from build123d import *

# Parameters (mm, degrees)
BOSS_EXTRUDE1_DEPTH            = 100
CUT_EXTRUDE3_DEPTH             = 202.556443707
CUT_EXTRUDE3_DEPTH_BACK        = 202.556443707
SKETCH4_4_R                    = 9.85
CUT_EXTRUDE4_DEPTH             = 3
CUT_EXTRUDE5_START             = 103
SKETCH4_6_R                    = 9.85
CUT_EXTRUDE5_DEPTH             = 103
CUT_EXTRUDE6_REACH             = 206.206
SKETCH5_R                      = 2.25
CUT_EXTRUDE6_DIRECTION_2_DEPTH = 205.205778567
CUT_EXTRUDE7_REACH             = 201.841
SKETCH6_R                      = 2.25
SKETCH7_W                      = 12
SKETCH7_H                      = 15
CUT_EXTRUDE8_DEPTH             = 197.242821038
FILLET3_R                      = 2.5
FILLET4_R                      = 2.5
FILLET6_R                      = 5
CUT_EXTRUDE11_REACH            = 198.243
SKETCH8_W                      = 41.5
SKETCH8_H                      = 5
CUT_EXTRUDE12_REACH            = 174.119
SKETCH9_R                      = 1.75


with BuildPart() as part:
    # Sketch1 → Boss-Extrude1 (new body)
    with BuildSketch(Plane.XY):
        Polygon((-10.600610125, 140), (-15.600610125, 140), (-15.600610125, -5), (94.399389875, -5), (94.399389875, 140), (89.399389875, 140), (89.399389875, 0), (-10.600610125, 0), align=None)
    extrude(amount=-BOSS_EXTRUDE1_DEPTH)

    # Sketch4 → Cut-Extrude3 (cut, two sides: drawn at the far end of the back side and taken through both)
    with BuildSketch(Plane.ZY.offset(-89.399389875).offset(-CUT_EXTRUDE3_DEPTH_BACK)):
        with BuildLine():
            ThreePointArc((-89.05, 45), (-82.05, 38), (-75.05, 45))
            Line((-75.05, 45), (-82.05, 45))
            Line((-82.05, 45), (-89.05, 45))
        make_face()
        with BuildLine():
            Line((-82.05, 45), (-75.05, 45))
            ThreePointArc((-75.05, 45), (-82.05, 52), (-89.05, 45))
            Line((-89.05, 45), (-82.05, 45))
        make_face()
        with BuildLine():
            ThreePointArc((-57, 45), (-50, 38), (-43, 45))
            Line((-43, 45), (-50, 45))
            Line((-50, 45), (-57, 45))
        make_face()
        with BuildLine():
            Line((-50, 45), (-43, 45))
            ThreePointArc((-43, 45), (-50, 52), (-57, 45))
            Line((-57, 45), (-50, 45))
        make_face()
        with BuildLine():
            ThreePointArc((-24.95, 45), (-17.95, 38), (-10.95, 45))
            Line((-10.95, 45), (-17.95, 45))
            Line((-17.95, 45), (-24.95, 45))
        make_face()
        with BuildLine():
            Line((-17.95, 45), (-10.95, 45))
            ThreePointArc((-10.95, 45), (-17.95, 52), (-24.95, 45))
            Line((-24.95, 45), (-17.95, 45))
        make_face()
    extrude(amount=CUT_EXTRUDE3_DEPTH + CUT_EXTRUDE3_DEPTH_BACK, mode=Mode.SUBTRACT)

    # Sketch4<4> → Cut-Extrude4 (cut)
    with BuildSketch(Plane.ZY.offset(-89.399389875)):
        with Locations((-50, 45)):
            Circle(SKETCH4_4_R)
        with Locations((-82.05, 45)):
            Circle(SKETCH4_4_R)
        with Locations((-17.95, 45)):
            Circle(SKETCH4_4_R)
    extrude(amount=-CUT_EXTRUDE4_DEPTH, mode=Mode.SUBTRACT)

    # Sketch4<6> → Cut-Extrude5 (cut)
    with BuildSketch(Plane.ZY.offset(-89.399389875).offset(CUT_EXTRUDE5_START)):
        with Locations((-50, 45)):
            Circle(SKETCH4_6_R)
        with Locations((-82.05, 45)):
            Circle(SKETCH4_6_R)
        with Locations((-17.95, 45)):
            Circle(SKETCH4_6_R)
    extrude(amount=-CUT_EXTRUDE5_DEPTH, mode=Mode.SUBTRACT)

    # Sketch5 → Cut-Extrude6 (cut, up to next)
    with BuildSketch(Plane.ZY.offset(15.600610125), mode=Mode.PRIVATE) as cut_extrude6_sk1:
        with Locations(Location((-78.75, 119.5, 0), (0, 0, 90))):
            Circle(SKETCH5_R)
    cut_extrude6_tool1 = extrude(cut_extrude6_sk1.sketch, amount=-CUT_EXTRUDE6_REACH, mode=Mode.PRIVATE) & part.part
    # Sketch5 → Cut-Extrude6 (cut, up to next)
    with BuildSketch(Plane.ZY.offset(15.600610125), mode=Mode.PRIVATE) as cut_extrude6_sk2:
        with Locations(Location((-21.25, 119.5, 0), (0, 0, 90))):
            Circle(SKETCH5_R)
    cut_extrude6_tool2 = extrude(cut_extrude6_sk2.sketch, amount=-CUT_EXTRUDE6_REACH, mode=Mode.PRIVATE) & part.part
    add(cut_extrude6_tool1.solids().sort_by_distance((-15.60061, 119.5, -78.75))[0], mode=Mode.SUBTRACT)
    add(cut_extrude6_tool2.solids().sort_by_distance((-15.60061, 119.5, -21.25))[0], mode=Mode.SUBTRACT)

    # Sketch5 → Cut-Extrude6 direction 2 (cut)
    with BuildSketch(Plane.ZY.offset(15.600610125)):
        with Locations(Location((-78.75, 119.5, 0), (0, 0, 90))):
            Circle(SKETCH5_R)
        with Locations(Location((-21.25, 119.5, 0), (0, 0, 90))):
            Circle(SKETCH5_R)
    extrude(amount=CUT_EXTRUDE6_DIRECTION_2_DEPTH, mode=Mode.SUBTRACT)

    # Sketch6 → Cut-Extrude7 (cut, up to next)
    with BuildSketch(Plane.XZ.offset(5), mode=Mode.PRIVATE) as cut_extrude7_sk1:
        with Locations(Location((71.899389875, -50, 0), (0, 0, 270))):
            Circle(SKETCH6_R)
    cut_extrude7_tool1 = extrude(cut_extrude7_sk1.sketch, amount=-CUT_EXTRUDE7_REACH, mode=Mode.PRIVATE) & part.part
    # Sketch6 → Cut-Extrude7 (cut, up to next)
    with BuildSketch(Plane.XZ.offset(5), mode=Mode.PRIVATE) as cut_extrude7_sk2:
        with Locations(Location((6.899389875, -50, 0), (0, 0, 270))):
            Circle(SKETCH6_R)
    cut_extrude7_tool2 = extrude(cut_extrude7_sk2.sketch, amount=-CUT_EXTRUDE7_REACH, mode=Mode.PRIVATE) & part.part
    add(cut_extrude7_tool1.solids().sort_by_distance((71.89939, -5, -50))[0], mode=Mode.SUBTRACT)
    add(cut_extrude7_tool2.solids().sort_by_distance((6.89939, -5, -50))[0], mode=Mode.SUBTRACT)

    # Sketch7 → Cut-Extrude8 (cut, through all)
    with BuildSketch(Plane(origin=(0, 0, 0), x_dir=(1, 0, 0), z_dir=(0, 1, 0))):
        Polygon((45.399389875, 100), (39.399389875, 100), (33.399389875, 100), (33.399389875, 85), (45.399389875, 85), align=None)
        with Locations((39.399389875, 7.5)):
            Rectangle(SKETCH7_W, SKETCH7_H)
    extrude(amount=-CUT_EXTRUDE8_DEPTH, mode=Mode.SUBTRACT)

    # Fillet3
    fillet3_edges = [part.edges().sort_by_distance(p)[0] for p in [
        (33.399389875, 0, -7.5),
        (33.399389875, -2.5, 0),
        (39.399389875, 0, -15),
        (33.399389875, -2.5, -15),
        (45.399389875, -5, -7.5),
        (45.399389875, -2.5, -15),
        (45.399389875, -2.5, 0),
        (33.399389875, -5, -7.5),
        (39.399389875, -5, -15),
        (45.399389875, 0, -7.5),
    ]]
    fillet(fillet3_edges, radius=FILLET3_R - 0.0001)  # a hair under: the kernel refuses the full size

    # Fillet4
    fillet4_edges = [part.edges().sort_by_distance(p)[0] for p in [
        (45.399389875, 0, -92.5),
        (45.399389875, -2.5, -100),
        (39.399389875, -5, -85),
        (45.399389875, -2.5, -85),
        (33.399389875, -5, -92.5),
        (33.399389875, -2.5, -85),
        (33.399389875, -2.5, -100),
        (45.399389875, -5, -92.5),
        (33.399389875, 0, -92.5),
        (39.399389875, 0, -85),
    ]]
    fillet(fillet4_edges, radius=FILLET4_R - 0.0001)  # a hair under: the kernel refuses the full size

    # Fillet6
    fillet6_edges = [part.edges().sort_by_distance(p)[0] for p in [
        (91.899389875, 140, -100),
        (-13.100610125, 140, -100),
        (-13.100610125, 140, 0),
        (91.899389875, 140, 0),
    ]]
    fillet(fillet6_edges, radius=FILLET6_R)

    # Sketch8 → Cut-Extrude11 (cut, up to next)
    with BuildSketch(Plane.XY, mode=Mode.PRIVATE) as cut_extrude11_sk1:
        with Locations((10.149389875, -2.5)):
            Rectangle(SKETCH8_W, SKETCH8_H)
    cut_extrude11_tool1 = extrude(cut_extrude11_sk1.sketch, amount=-CUT_EXTRUDE11_REACH, mode=Mode.PRIVATE) & part.part
    # Sketch8 → Cut-Extrude11 (cut, up to next)
    with BuildSketch(Plane.XY, mode=Mode.PRIVATE) as cut_extrude11_sk2:
        Polygon((-10.600610125, 135), (-10.600610125, 0), (30.899389875, 0), (30.899389875, -5), (94.399389875, -5), (94.399389875, 140), (-10.600610125, 140), align=None)
    cut_extrude11_tool2 = extrude(cut_extrude11_sk2.sketch, amount=-CUT_EXTRUDE11_REACH, mode=Mode.PRIVATE) & part.part
    add(cut_extrude11_tool1.solids().sort_by_distance((10.14939, -2.5, 0))[0], mode=Mode.SUBTRACT)
    add(cut_extrude11_tool2.solids().sort_by_distance((42.338086, 68.467205, 0))[0], mode=Mode.SUBTRACT)

    # Sketch9 → Cut-Extrude12 (cut, up to next)
    with BuildSketch(Plane(origin=(-10.600610125, 0, 0), x_dir=(0, 0, -1), z_dir=(1, 0, 0)), mode=Mode.PRIVATE) as cut_extrude12_sk1:
        with Locations(Location((70, 8.5, 0), (0, 0, 90))):
            Circle(SKETCH9_R)
    cut_extrude12_tool1 = extrude(cut_extrude12_sk1.sketch, amount=-CUT_EXTRUDE12_REACH, mode=Mode.PRIVATE) & part.part
    # Sketch9 → Cut-Extrude12 (cut, up to next)
    with BuildSketch(Plane(origin=(-10.600610125, 0, 0), x_dir=(0, 0, -1), z_dir=(1, 0, 0)), mode=Mode.PRIVATE) as cut_extrude12_sk2:
        with Locations(Location((50, 8.5, 0), (0, 0, 90))):
            Circle(SKETCH9_R)
    cut_extrude12_tool2 = extrude(cut_extrude12_sk2.sketch, amount=-CUT_EXTRUDE12_REACH, mode=Mode.PRIVATE) & part.part
    # Sketch9 → Cut-Extrude12 (cut, up to next)
    with BuildSketch(Plane(origin=(-10.600610125, 0, 0), x_dir=(0, 0, -1), z_dir=(1, 0, 0)), mode=Mode.PRIVATE) as cut_extrude12_sk3:
        with Locations(Location((30, 8.5, 0), (0, 0, 90))):
            Circle(SKETCH9_R)
    cut_extrude12_tool3 = extrude(cut_extrude12_sk3.sketch, amount=-CUT_EXTRUDE12_REACH, mode=Mode.PRIVATE) & part.part
    add(cut_extrude12_tool1.solids().sort_by_distance((-10.60061, 8.5, -70))[0], mode=Mode.SUBTRACT)
    add(cut_extrude12_tool2.solids().sort_by_distance((-10.60061, 8.5, -50))[0], mode=Mode.SUBTRACT)
    add(cut_extrude12_tool3.solids().sort_by_distance((-10.60061, 8.5, -30))[0], mode=Mode.SUBTRACT)


solid = part.part
For this review, take the finished solid that the model builds, in its own axes (mm). A direction names the side the tool comes from. Give positions to 0.01 mm unless a question says otherwise; leave off trailing zeros. Loops run counter-clockwise (first coordinate to the right, second up) from the corner with the lowest first, then second, coordinate; pieces in that order, holes last.
Item 1: Take a section at C-C, the plane z = -70. State the section outline as (x, y) points.
Item 2: Take a section at B-B, the plane x = -11.4. Give the number of separate pieces and of enclosed holes in the cut face, and give its area (3 significant figures).
Item 3: Tool access review of faces 5 (the cylindrical face through (-13.07, 8.12, -71.71)), 6 (the flat face through (-13.601, 52, -80)): name each direction out of +Z, -Z, +X, -X, +Y, -Y from which nothing blocks a thin tool from reaching the whole face with its end or side.
Item 4: For line 1 along Z through (x, y) = (-11.95, 119.5); line 2 along Z through (x, y) = (-14.85, 45); line 3 along Y through (x, z) = (-12.25, -82.05), list the stretches that pass through material, from the lowest coordinate up.
Item 5: Insertion check: pin 1 (17.5 mm diameter, centred on y = 45, z = -82.05, fed in from +X). The pin has a flat end and moves straight along its axis. Give the tip position at first contact, or say it passes through.
Item 6: Take a section at A-A, the plane y = 119.5. State the section outline as (x, z) points.
Item 7: Take a section at D-D, the plane y = 45. State the section outline as (x, z) points, and give its area (3 significant figures).
Item 8: Draft analysis for pull direction Z (two halves, no side actions). For faces 1 (the flat face through (-13, -5, -49)), 2 (the cylindrical face through (-13.14, 121.58, -77.89)), 3 (the cylindrical face through (-13.07, 9.31, -31.55)), 4 (the cylindrical face through (-13, 138, -99)), state which applies: +Z half, -Z half, draft (parallel to the pull), parting line (faces both ways), or undercut.
Calculated:
1. outline: (-15.6, -5) - (-10.6, -5) - (-10.6, 6.75) - (-15.6, 6.75) - close; (-15.6, 10.25) - (-10.6, 10.25) - (-10.6, 140) - (-15.6, 140) - close
2. separate pieces: 1
2. enclosed holes: 8
2. area: 13,500 mm2
3. face 5: +X, -X
3. face 6: +X
4. line 1: z = -100 to -81, -76.5 to -23.5, -19 to 0
4. line 2: z = -100 to -89.05, -75.05 to -57, -43 to -24.95, -10.95 to 0
4. line 3: y = -5 to 35.15, 54.85 to 140
5. pin 1: stops at x = -13.6
6. outline: (-15.6, -100) - (-10.6, -100) - (-10.6, -81) - (-15.6, -81) - close; (-15.6, -76.5) - (-10.6, -76.5) - (-10.6, -23.5) - (-15.6, -23.5) - close; (-15.6, -19) - (-10.6, -19) - (-10.6, 0) - (-15.6, 0) - close
7. outline: (-15.6, -100) - (-10.6, -100) - (-10.6, -91.9) - (-13.6, -91.9) - (-13.6, -89.05) - (-15.6, -89.05) - close; (-15.6, -75.05) - (-13.6, -75.05) - (-13.6, -72.2) - (-10.6, -72.2) - (-10.6, -59.85) - (-13.6, -59.85) - (-13.6, -57) - (-15.6, -57) - close; (-15.6, -43) - (-13.6, -43) - (-13.6, -40.15) - (-10.6, -40.15) - (-10.6, -27.8) - (-13.6, -27.8) - (-13.6, -24.95) - (-15.6, -24.95) - close; (-15.6, -10.95) - (-13.6, -10.95) - (-13.6, -8.1) - (-10.6, -8.1) - (-10.6, 0) - (-15.6, 0) - close
7. area: 239 mm2
8. face 1: draft
8. face 2: undercut
8. face 3: undercut
8. face 4: -Z half
